```python
from build123d import *

# Parameters (mm, degrees)
F0_R     = 32.5
F1_DEPTH = 3
F2_R     = 22.5
F3_DEPTH = 20
F4_R     = 20.5
F5_DEPTH = 23.001
F6_R     = 3.05
F6_R_2   = 1
F7_DEPTH = 3.001


with BuildPart() as f1:
    # F0 (on Front) → F1 (new body)
    with BuildSketch(Plane.XZ):
        Circle(F0_R)
    extrude(amount=F1_DEPTH)

    # F2 (on face) → F3 (join)
    with BuildSketch(Plane.XZ.offset(3)):
        Circle(F2_R)
    extrude(amount=F3_DEPTH)

    # F4 (on face) → F5 (cut, through all)
    with BuildSketch(Plane.XZ.offset(23)):
        Circle(F4_R)
    extrude(amount=-F5_DEPTH, mode=Mode.SUBTRACT)

    # F6 (on face) → F7 (cut, through all)
    with BuildSketch(Plane.XZ.offset(3)):
        with Locations((27.5, 0)):
            Circle(F6_R)
        with Locations((-27.5, 0)):
            Circle(F6_R)
        with Locations((0, 22.5)):
            Circle(F6_R_2)
    extrude(amount=-F7_DEPTH, mode=Mode.SUBTRACT)


solid = f1.part
```
Model file for the job. Use its own axes, mm. A direction names the side the tool comes from. Coordinates: 2 decimals unless noted, no trailing zeros. Loops run counter-clockwise (first coordinate to the right, second up) from the corner with the lowest first, then second, coordinate; pieces in that order, holes last. Notation, with made-up numbers: (-9.75, 8.25) -> (-2.75, 8.25) arc R15 ccw to (-2.75, 12.25) -> close; hole circle Ø7 at (48, 68.5). An arc over 180 degrees is marked (long way). Answer as a JSON object with one key per item and string values.
Q1. Cut at C-C (x = -27.5). List the corners of the cut face in (y, z), and give its area (3 significant figures).
Report:
{"outline": "(-3, -17.32) -> (0, -17.32) -> (0, -3.05) -> (-3, -3.05) -> close; (-3, 3.05) -> (0, 3.05) -> (0, 17.32) -> (-3, 17.32) -> close", "area": "85.6 mm2"}
Q2. Cut at D-D (z = 0). List the corners of the cut face in (x, y).
Report:
{"outline": "(-32.5, -3) -> (-30.55, -3) -> (-30.55, 0) -> (-32.5, 0) -> close; (-24.45, -3) -> (-22.5, -3) -> (-22.5, -23) -> (-20.5, -23) -> (-20.5, 0) -> (-24.45, 0) -> close; (20.5, -23) -> (22.5, -23) -> (22.5, -3) -> (24.45, -3) -> (24.45, 0) -> (20.5, 0) -> close; (30.55, -3) -> (32.5, -3) -> (32.5, 0) -> (30.55, 0) -> close"}
Q3. Probe probe 1 along Z at (x, y) = (0, -1.6); probe 2 along Y at (x, z) = (13.5, 24.5); probe 3 along Z at (x, y) = (27.5, -1.4). List the from-to ranges inside material, lowest first.
Report:
{"probe 1": "z = -32.5 to -20.5, 20.5 to 21.5, 23.5 to 32.5", "probe 2": "y = -3 to 0", "probe 3": "z = -17.32 to -3.05, 3.05 to 17.32"}
Q4. 3-axis set-ups, long thin cutter, end or side, ignore diameter. For faces 4 (the cylindrical face through (31, -1.48, 9.76)), 5 (the flat face through (7, -3, 22)): which of +Z, -Z, +X, -X, +Y, -Y reach the whole face in a straight line?
Report:
{"face 4": "+Y, -Y", "face 5": "-Y"}
Q5. Pull direction X, two halves, no side cores. Call faces 1 (the cylindrical face through (0.46, -1.52, 21.61)), 2 (the flat face through (9.9, -23, -18.2)), 3 (the cylindrical face through (10.382, -12.86, -19.961)): released by +X, released by -X, zero draft, split by the parting line, or undercut.
Report:
{"face 1": "undercut", "face 2": "zero draft", "face 3": "split by the parting line"}
Q6. Cut at A-A (x = 0). List the corners of the cut face in (y, z).
Report:
{"outline": "(-23, -22.5) -> (-3, -22.5) -> (-3, -32.5) -> (0, -32.5) -> (0, -20.5) -> (-23, -20.5) -> close; (-23, 20.5) -> (0, 20.5) -> (0, 21.5) -> (-3, 21.5) -> (-3, 22.5) -> (-23, 22.5) -> close; (-3, 23.5) -> (0, 23.5) -> (0, 32.5) -> (-3, 32.5) -> close"}
Q7. Cut at B-B (z = 19). List the corners of the cut face in (x, y).
Report:
{"outline": "(-26.37, -3) -> (-12.05, -3) -> (-12.05, -23) -> (-7.7, -23) -> (-7.7, 0) -> (-26.37, 0) -> close; (7.7, -23) -> (12.05, -23) -> (12.05, -3) -> (26.37, -3) -> (26.37, 0) -> (7.7, 0) -> close"}
Q8. Flat gauge pins, fed straight in: P1, Ø3, axis at y = -14.5, z = -10.5, coming from the +X side; P2, Ø1.5, axis at x = 15.5, y = -11.5, coming from the -Z side; P3, Ø12, axis at x = -16.5, y = -20.5, coming from the -Z side; P4, Ø3.5, axis at x = 27.5, z = 0, coming from the -Y side. Where does each tip first touch, or does it go through?
Report:
{"P1": "stops at x = 20.62", "P2": "stops at z = -16.99", "P3": "stops at z = -19.9", "P4": "passes through"}
